Could you check a few things on this model? Use its own coordinates, in mm. Face numbers are marked on the shaded views. Round coordinates to 2 decimals unless told otherwise and drop trailing zeros. Loops run counter-clockwise (first coordinate to the right, second up) from the corner with the lowest first, then second, coordinate; pieces in that order, holes last. Notation, with made-up numbers: (62, -31.5) -> (72, -31.5) arc R35 cw to (72, 3.5) -> close; hole circle Ø8 at (-30, -12.5). An arc over 180 degrees is marked (long way). Write each question's results on one line, items separated by ' | '.
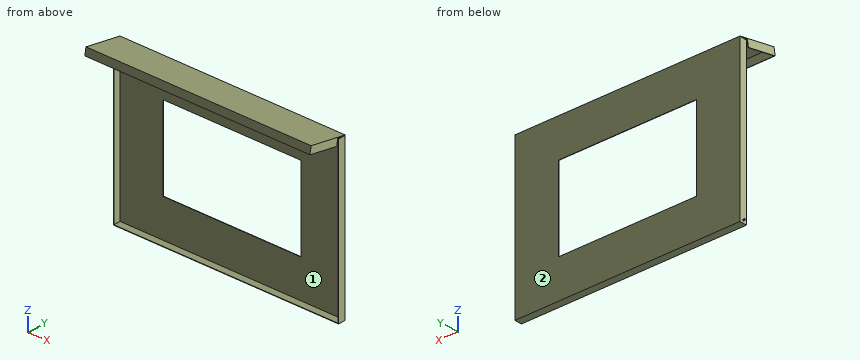
from build123d import *

# Parameters (mm, degrees)
CROQUIS1_W              = 490
CROQUIS1_H              = 345.25
SALIENTE_EXTRUIR1_DEPTH = 1
CROQUIS2_W              = 300
CROQUIS2_H              = 180
CORTAR_EXTRUIR1_DEPTH   = 2
SALIENTE_EXTRUIR2_DEPTH = 490
SALIENTE_EXTRUIR3_DEPTH = 15
SALIENTE_EXTRUIR4_DEPTH = 15
CROQUIS6_R              = 1.5
SALIENTE_EXTRUIR5_DEPTH = 3


with BuildPart() as part:
    # Croquis1 → Saliente-Extruir1 (new body)
    with BuildSketch(Plane(origin=(0, 0, 0), x_dir=(1, 0, 0), z_dir=(0, 1, 0))):
        Rectangle(CROQUIS1_W, CROQUIS1_H)
    extrude(amount=SALIENTE_EXTRUIR1_DEPTH)

    # Croquis2 → Cortar-Extruir1 (cut, through all)
    with BuildSketch(Plane(origin=(0, 1, 0), x_dir=(1, 0, 0), z_dir=(0, 1, 0))):
        Rectangle(CROQUIS2_W, CROQUIS2_H)
    extrude(amount=-CORTAR_EXTRUIR1_DEPTH, mode=Mode.SUBTRACT)

    # Croquis3 → Saliente-Extruir2 (add, through all)
    with BuildSketch(Plane(origin=(245, 0, 0), x_dir=(0, 0, -1), z_dir=(1, 0, 0))):
        Polygon((-172.625, 1), (-187.211446924, -81.723851253), (-186.226639171, -81.897499431), (-171.609573388, 1), align=None)
    extrude(amount=-SALIENTE_EXTRUIR2_DEPTH)

    # Croquis4 → Saliente-Extruir3 (add)
    with BuildSketch(Plane.XZ):
        Polygon((-245, -172.625), (-245, 171.785900369), (-244, 171.785900369), (-244, -171.625), (244, -171.625), (244, 171.785900369), (245, 171.785900369), (245, -172.625), align=None)
    extrude(amount=SALIENTE_EXTRUIR3_DEPTH)

    # Croquis5 → Saliente-Extruir4 (add)
    with BuildSketch(Plane(origin=(0, 29.377119133, 166.60592165), x_dir=(-1, 0, 0), z_dir=(0, -0.173648178, -0.984807753))):
        Polygon((-244, -111.991208917), (-244, -46.991208917), (-245, -46.991208917), (-245, -112.991208917), (245, -112.991208917), (245, -46.991208917), (244, -46.991208917), (244, -111.991208917), align=None)
    extrude(amount=SALIENTE_EXTRUIR4_DEPTH)

    # Croquis6 → Saliente-Extruir5 (add)
    with BuildSketch(Plane.ZY.offset(245)):
        with Locations((-166.625, -7)):
            Circle(CROQUIS6_R)
    extrude(amount=SALIENTE_EXTRUIR5_DEPTH)


solid = part.part
1) If we mould it in two halves opening along X, with no side actions, what happens to the marked faces 1 and 2? For each: released by +X, released by -X, zero draft, split by the parting line, or undercut.
Model answer:
face 1: undercut | face 2: zero draft
2) I want a section at D-D, the plane y = -49.5. Write out the boundary of the cut face in (x, z), plus the area to 3 significant figures.
Model answer:
outline: (-245, 165.28) -> (-244, 165.28) -> (-244, 180.51) -> (244, 180.51) -> (244, 165.28) -> (245, 165.28) -> (245, 181.53) -> (-245, 181.53) -> close | area: 528 mm2
3) I want a section at B-B, the plane z = -18. Write out the boundary of the cut face in (x, y), plus the area to 3 significant figures.
Model answer:
outline: (-245, -15) -> (-244, -15) -> (-244, 0) -> (-150, 0) -> (-150, 1) -> (-245, 1) -> close; (150, 0) -> (244, 0) -> (244, -15) -> (245, -15) -> (245, 1) -> (150, 1) -> close | area: 220 mm2
4) I want a section at C-C, the plane x = -163. Write out the boundary of the cut face in (y, z) (3 decimals).
Model answer:
outline: (-84.502, 171.455) -> (-83.517, 171.281) -> (-80.913, 186.053) -> (0, 171.786) -> (0, -171.625) -> (-15, -171.625) -> (-15, -172.625) -> (1, -172.625) -> (1, 172.625) -> (-81.724, 187.211) -> close
5) I need wall thicknesses on line 1 (X direction, y = -9.5, z = -130.5); line 2 (Y direction, x = 105.5, z = -117); line 3 (Z direction, x = -64, y = -9) (3 decimals). Which ranges of each line are inside material? Lowest first, please.
Model answer:
line 1: x = -245 to -244, 244 to 245 | line 2: y = 0 to 1 | line 3: z = -172.625 to -171.625, 173.373 to 174.388
6) I'm going to push flat-ended pins straight in: pin 1 (12 mm diameter, centred on x = -63, y = -4.5, fed in from +Z); pin 2 (12 mm diameter, centred on x = -118.5, y = -55.5, fed in from -Z); pin 3 (10 mm diameter, centred on x = -31, z = -129, fed in from -Y); pin 4 (8 mm diameter, centred on y = -22, z = 100.5, fed in from -X). Where does each tip first touch, or does it pass through?
Model answer:
pin 1: stops at z = 174.65 | pin 2: stops at z = 180.51 | pin 3: stops at y = 0 | pin 4: passes through
7) I want a section at A-A, the plane x = 71.5. Write out the boundary of the cut face in (y, z) (3 decimals), plus the area to 3 significant figures.
Model answer:
outline: (-84.502, 171.455) -> (-83.517, 171.281) -> (-80.913, 186.053) -> (0, 171.786) -> (0, 90) -> (1, 90) -> (1, 172.625) -> (-81.724, 187.211) -> close; (-15, -172.625) -> (1, -172.625) -> (1, -90) -> (0, -90) -> (0, -171.625) -> (-15, -171.625) -> close | area: 278 mm2
